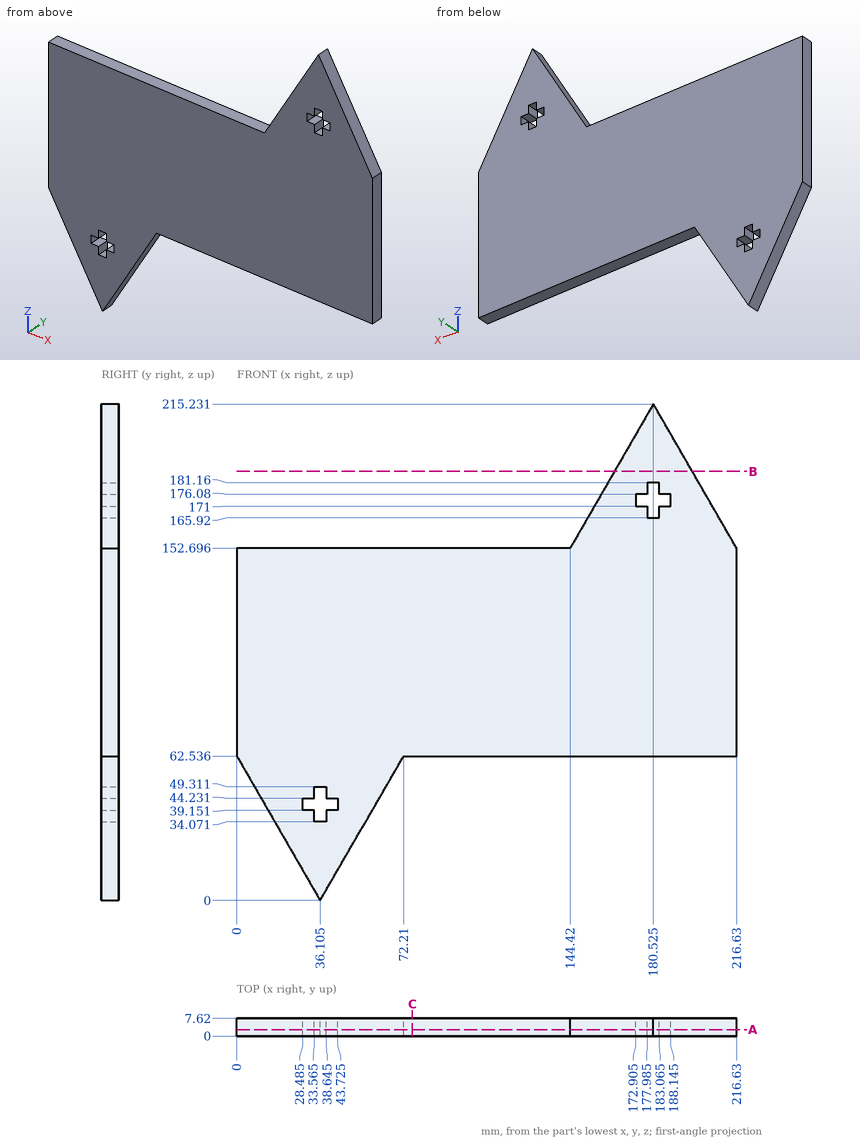
Check sheet for the drawn part. Datum: minimum x, y, z corner. Units: mm. Coordinates: 2 decimals unless noted, no trailing zeros. Order: outer loops, then holes, each group sorted by start corner. A loop starts at its lowest first (then second) coordinate and runs counter-clockwise, first axis right, second up. Notation, with made-up numbers: (86.25, 19.5) -> (111.25, 19.5) arc R21 cw to (111.25, 36.5) -> close; hole circle Ø5 at (89.25, 63). An arc over 180 degrees is marked (long way). Use a Markdown table: item, result. Add a question column.
1. Go/stop test with flat-tipped pins: pin 1 Ø2.5 at (x, y) = (181.5, 5) entering from -Z; pin 2 Ø4 at (y, z) = (3.5, 174) entering from +X (1 decimal); pin 3 Ø2.5 at (y, z) = (4, 36.5) entering from +X. Record where each tip stops, or that it passes through.
2. Cross-section at A-A (y = 2.75). Give the number of separate pieces and of enclosed holes in the cut face, and give its area (3 significant figures).
3. Cross-section at C-C (x = 76). Enter the section's corners in (y, z) (1 decimal).
4. Cross-section at B-B (z = 186). Enter the section's corners in (x, y).
5. Material ranges on L1, parallel to Z at x = 129.5, y = 3.75 (1 decimal); L2, parallel to Z at x = 170.5, y = 6.25 (1 decimal); L3, parallel to X at y = 2.25, z = 190, recorded low to high.
Filled sheet:
| question | item | result |
|---|---|---|
| 1 | pin 1 | z = 62.54 |
| 1 | pin 2 | x = 205.5 |
| 1 | pin 3 | x = 57.9 |
| 2 | separate pieces | 1 |
| 2 | enclosed holes | 2 |
| 2 | area | 23,800 mm2 |
| 3 | outline | (0, 62.5) -> (7.6, 62.5) -> (7.6, 152.7) -> (0, 152.7) -> close |
| 4 | outline | (163.65, 0) -> (197.4, 0) -> (197.4, 7.62) -> (163.65, 7.62) -> close |
| 5 | L1 | 62.5 to 152.7 |
| 5 | L2 | 62.5 to 197.9 |
| 5 | L3 | 165.96 to 195.09 |
